For this review, take the finished solid that the model builds, in its own axes (mm). Coordinates: 2 decimals unless noted, no trailing zeros. Loops run counter-clockwise (first coordinate to the right, second up) from the corner with the lowest first, then second, coordinate; pieces in that order, holes last.
```python
from build123d import *

# Parameters (mm, degrees)
EXTRUDE_1_DEPTH        = 1000
SKETCH_2_R             = 1.5
CUT_EXTRUDE_1_DEPTH    = 20
SKETCH_3_R             = 3
CUT_EXTRUDE_2_DEPTH    = 4.5
PATTERN_LINEAR_1_COUNT = 25
PATTERN_LINEAR_1_PITCH = 40
CUT_EXTRUDE_4_DEPTH    = 80
CUT_EXTRUDE_5_DEPTH    = 80
EXTRUDE_START          = 15
EXTRUDE_2_DEPTH        = 15
CUT_EXTRUDE_START      = -30
CUT_EXTRUDE_8_DEPTH    = 30


with BuildPart() as part:
    # 草图1 → 凸台-拉伸1 (new body)
    with BuildSketch(Plane.XY):
        with BuildLine():
            Line((-7.643186957, 0.234233912), (-7.643186957, -4.365766088))
            Line((-7.643186957, -4.365766088), (-7.243186957, -4.765766088))
            Line((-7.243186957, -4.765766088), (6.956813043, -4.765766088))
            Line((6.956813043, -4.765766088), (7.356813043, -4.365766088))
            Line((7.356813043, -4.365766088), (7.356813043, 0.234233912))
            ThreePointArc((7.356813043, 0.234233912), (6.296152871, 0.67357374), (5.856813043, 1.734233912))
            ThreePointArc((5.856813043, 1.734233912), (6.296152871, 2.794894084), (7.356813043, 3.234233912))
            Line((7.356813043, 3.234233912), (7.356813043, 4.834233912))
            Line((7.356813043, 4.834233912), (6.956813043, 5.234233912))
            Line((6.956813043, 5.234233912), (-7.243186957, 5.234233912))
            Line((-7.243186957, 5.234233912), (-7.643186957, 4.834233912))
            Line((-7.643186957, 4.834233912), (-7.643186957, 3.234233912))
            ThreePointArc((-7.643186957, 3.234233912), (-6.143186957, 1.734233912), (-7.643186957, 0.234233912))
        make_face()
    extrude(amount=EXTRUDE_1_DEPTH)

    # 草图2 → 切除-拉伸1 (cut)
    with BuildSketch(Plane(origin=(0, 5.234233912, 0), x_dir=(1, 0, 0), z_dir=(0, 1, 0))):
        with Locations(Location((0, -20, 0), (0, 0, 270))):
            Circle(SKETCH_2_R)
    cut_extrude_1 = extrude(amount=-CUT_EXTRUDE_1_DEPTH, mode=Mode.SUBTRACT)

    # 草图3 → 切除-拉伸2 (cut)
    with BuildSketch(Plane(origin=(0, 5.234233912, 0), x_dir=(1, 0, 0), z_dir=(0, 1, 0))):
        with Locations(Location((0, -20, 0), (0, 0, 270))):
            Circle(SKETCH_3_R)
    cut_extrude_2 = extrude(amount=-CUT_EXTRUDE_2_DEPTH, mode=Mode.SUBTRACT)

    # 阵列(线性)1: 切除-拉伸1, 切除-拉伸2 ×25
    with Locations(*[(0, 0, i * PATTERN_LINEAR_1_PITCH) for i in range(1, PATTERN_LINEAR_1_COUNT)]):
        add(cut_extrude_1, mode=Mode.SUBTRACT)
        add(cut_extrude_2, mode=Mode.SUBTRACT)

    # 草图6 → 切除-拉伸4 (cut)
    with BuildSketch(Plane(origin=(0, 0, 0), x_dir=(-1, 0, 0), z_dir=(0, 0, -1))):
        with BuildLine():
            Line((7.643186957, 3.234233912), (7.643186957, 4.834233912))
            Line((7.643186957, 4.834233912), (7.243186957, 5.234233912))
            Line((7.243186957, 5.234233912), (-6.956813043, 5.234233912))
            Line((-6.956813043, 5.234233912), (-7.356813043, 4.834233912))
            Line((-7.356813043, 4.834233912), (-7.356813043, 3.234233912))
            ThreePointArc((-7.356813043, 3.234233912), (-5.856813043, 1.734233912), (-7.356813043, 0.234233912))
            Line((-7.356813043, 0.234233912), (-7.356813043, -4.365766088))
            Line((-7.356813043, -4.365766088), (-6.956813043, -4.765766088))
            Line((-6.956813043, -4.765766088), (7.243186957, -4.765766088))
            Line((7.243186957, -4.765766088), (7.643186957, -4.365766088))
            Line((7.643186957, -4.365766088), (7.643186957, 0.234233912))
            ThreePointArc((7.643186957, 0.234233912), (6.143186957, 1.734233912), (7.643186957, 3.234233912))
        make_face()
    extrude(amount=-CUT_EXTRUDE_4_DEPTH, mode=Mode.SUBTRACT)

    # 草图7 → 切除-拉伸5 (cut)
    with BuildSketch(Plane(origin=(0, 0, 80), x_dir=(-1, 0, 0), z_dir=(0, 0, -1))):
        with BuildLine():
            Line((7.643186957, 3.234233912), (7.643186957, 4.834233912))
            Line((7.643186957, 4.834233912), (7.243186957, 5.234233912))
            Line((7.243186957, 5.234233912), (-6.956813043, 5.234233912))
            Line((-6.956813043, 5.234233912), (-7.356813043, 4.834233912))
            Line((-7.356813043, 4.834233912), (-7.356813043, 3.234233912))
            ThreePointArc((-7.356813043, 3.234233912), (-5.856813043, 1.734233912), (-7.356813043, 0.234233912))
            Line((-7.356813043, 0.234233912), (-7.356813043, -4.365766088))
            Line((-7.356813043, -4.365766088), (-6.956813043, -4.765766088))
            Line((-6.956813043, -4.765766088), (7.243186957, -4.765766088))
            Line((7.243186957, -4.765766088), (7.643186957, -4.365766088))
            Line((7.643186957, -4.365766088), (7.643186957, 0.234233912))
            ThreePointArc((7.643186957, 0.234233912), (6.143186957, 1.734233912), (7.643186957, 3.234233912))
        make_face()
    extrude(amount=-CUT_EXTRUDE_5_DEPTH, mode=Mode.SUBTRACT)

    # 草图10 → 凸台-拉伸2 (add)
    with BuildSketch(Plane(origin=(0, 0, 160), x_dir=(-1, 0, 0), z_dir=(0, 0, -1)).offset(EXTRUDE_START)):
        with BuildLine():
            Line((7.643186957, 3.234233912), (7.643186957, 4.834233912))
            Line((7.643186957, 4.834233912), (7.243186957, 5.234233912))
            Line((7.243186957, 5.234233912), (-6.956813043, 5.234233912))
            Line((-6.956813043, 5.234233912), (-7.356813043, 4.834233912))
            Line((-7.356813043, 4.834233912), (-7.356813043, 3.234233912))
            ThreePointArc((-7.356813043, 3.234233912), (-5.856813043, 1.734233912), (-7.356813043, 0.234233912))
            Line((-7.356813043, 0.234233912), (-7.356813043, -4.365766088))
            Line((-7.356813043, -4.365766088), (-6.956813043, -4.765766088))
            Line((-6.956813043, -4.765766088), (7.243186957, -4.765766088))
            Line((7.243186957, -4.765766088), (7.643186957, -4.365766088))
            Line((7.643186957, -4.365766088), (7.643186957, 0.234233912))
            ThreePointArc((7.643186957, 0.234233912), (6.143186957, 1.734233912), (7.643186957, 3.234233912))
        make_face()
    extrude(amount=-EXTRUDE_2_DEPTH)

    # 草图11 → 切除-拉伸8 (cut)
    with BuildSketch(Plane.XY.offset(1000).offset(CUT_EXTRUDE_START)):
        with BuildLine():
            Line((-7.643186957, 0.234233912), (-7.643186957, -4.365766088))
            Line((-7.643186957, -4.365766088), (-7.243186957, -4.765766088))
            Line((-7.243186957, -4.765766088), (6.956813043, -4.765766088))
            Line((6.956813043, -4.765766088), (7.356813043, -4.365766088))
            Line((7.356813043, -4.365766088), (7.356813043, 0.234233912))
            ThreePointArc((7.356813043, 0.234233912), (5.856813043, 1.734233912), (7.356813043, 3.234233912))
            Line((7.356813043, 3.234233912), (7.356813043, 4.834233912))
            Line((7.356813043, 4.834233912), (6.956813043, 5.234233912))
            Line((6.956813043, 5.234233912), (-7.243186957, 5.234233912))
            Line((-7.243186957, 5.234233912), (-7.643186957, 4.834233912))
            Line((-7.643186957, 4.834233912), (-7.643186957, 3.234233912))
            ThreePointArc((-7.643186957, 3.234233912), (-6.143186957, 1.734233912), (-7.643186957, 0.234233912))
        make_face()
    extrude(amount=CUT_EXTRUDE_8_DEPTH, mode=Mode.SUBTRACT)


solid = part.part
```
Q1. Consider section A-A (z = 326.5). State the section outline as (x, y) points, then the cut area to 3 significant figures.
Q2. For pin 1 Ø6.5 at (x, z) = (1, 179.5) entering from +Y; pin 2 Ø1.8 at (x, z) = (-0.5, 821.5) entering from +Y, all flat-tipped, find the tip position at first contact; note any pin that passes through.
Q3. Wall thickness on probe 1 along Y at (x, z) = (-7, 702.5); probe 2 along X at (y, z) = (-1.75, 260); probe 3 along Y at (x, z) = (6.5, 559.5): over which ranges is each line inside the solid? List them lowest first.
Model answer:
1. outline: (-7.64, -4.37) - (-7.24, -4.77) - (6.96, -4.77) - (7.36, -4.37) - (7.36, 0.23) arc R1.5 cw to (7.36, 3.23) - (7.36, 4.83) - (6.96, 5.23) - (-7.24, 5.23) - (-7.64, 4.83) - (-7.64, 3.23) arc R1.5 cw to (-7.64, 0.23) - close
1. area: 143 mm2
2. pin 1: stops at y = 5.23
2. pin 2: stops at y = 0.73
3. probe 1: y = -4.77 to 0.38, 3.09 to 5.23
3. probe 2: x = -7.64 to -1.5, 1.5 to 7.36
3. probe 3: y = -4.77 to 0.5, 2.97 to 5.23
